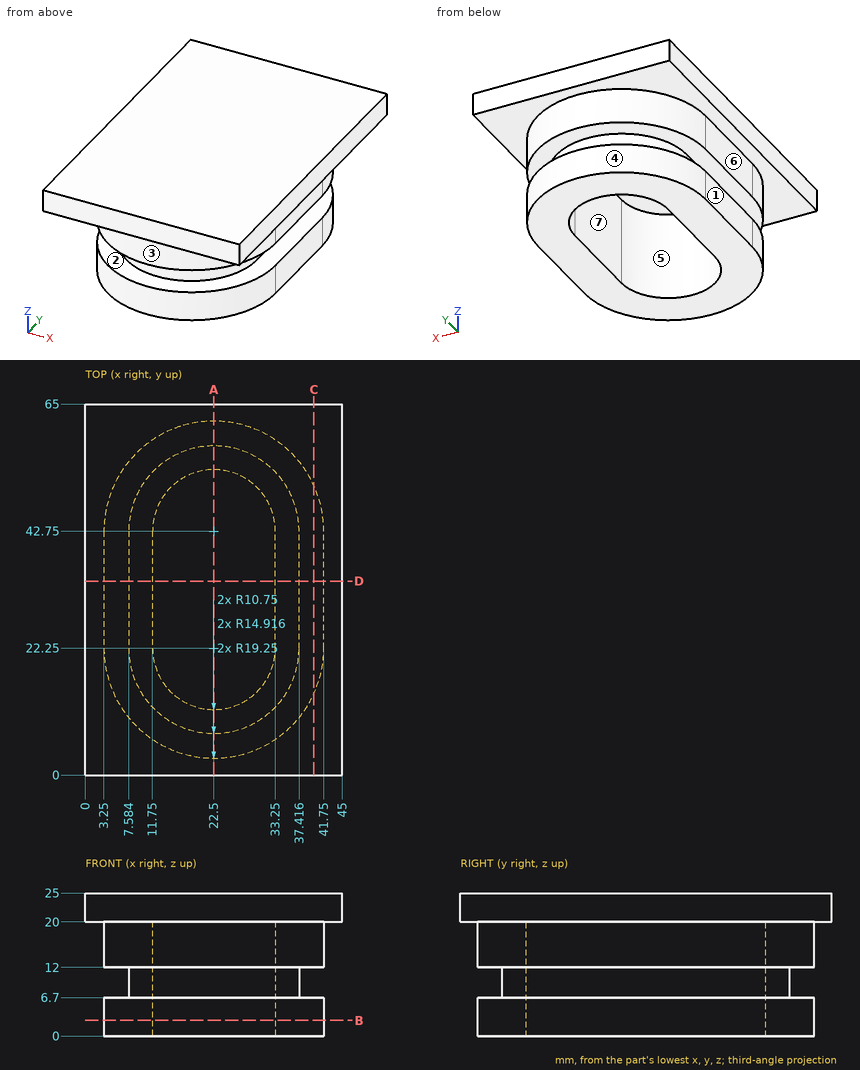
Could you check a few things on this drawing? It's one solid part, dimensions in mm from its lowest x, y, z. A direction names the side the tool comes from. Give positions to 0.01 mm unless a question says otherwise; leave off trailing zeros. Order: outer loops, then holes, each group sorted by start corner. A loop starts at its lowest first (then second) coordinate and runs counter-clockwise, first axis right, second up. Notation, with made-up numbers: (-1.75, -19.75) - (40.25, -19.75) arc R24 ccw to (40.25, -1.75) - close; hole circle Ø4 at (23, 67). An arc over 180 degrees is marked (long way). Return JSON: item names as keys, results as strings. Group by question number.
Q1. Will these pins go through, and if not, where does the flat tip stop? pin 1 Ø7.5 at (y, z) = (32, 2) entering from -X; pin 2 Ø4 at (y, z) = (34.5, 15) entering from +X; pin 3 Ø10 at (x, y) = (17, 51) entering from -Z; pin 4 Ø10 at (y, z) = (56.5, 13) entering from +X.
Q2. Thinking about a two-plate mould opening in X: for the marked faces 4, 5, 6 and 7, which applies, pulls with the +X half, pulls with the -X half, needs draft (parallel to the pull), parting line crosses it, or undercut?
Q3. Suppose I cut it at B-B, the plane z = 2.75. Please give me the cut outline in (x, y).
Q4. Suppose I cut it at C-C, the plane x = 40. Please give me the cut outline in (y, z), and give its area (3 significant figures).
Q5. Which directions (+Z, -Z, +X, -X, +Y, -Y) give clear straight access to the entire face, cutting with the end or side of a thin tool? Please do the marked faces 1, 2 and 3.
Q6. Suppose I cut it at D-D, the plane y = 34. Please give me the cut outline in (x, z), and give its area (3 significant figures).
Q7. Suppose I cut it at A-A, the plane x = 22.5. Please give me the cut outline in (y, z).
Q8. Please list where these lines run through material, in increasing order: line 1 along Y through (x, z) = (23, 16.25); line 2 along X through (y, z) = (22, 19.25). Write a range as [from, to].
Resolved:
{
 "1": {"pin 1": "stops at x = 3.25", "pin 2": "stops at x = 41.75", "pin 3": "stops at z = 0", "pin 4": "stops at x = 39.65"},
 "2": {"face 4": "parting line crosses it", "face 5": "undercut", "face 6": "pulls with the -X half", "face 7": "undercut"},
 "3": {"outline": "(3.25, 22.25) arc R19.25 ccw to (41.75, 22.25) - (41.75, 42.75) arc R19.25 ccw to (3.25, 42.75) - close; hole (11.75, 22.25) arc R10.75 ccw to (33.25, 22.25) - (33.25, 42.75) arc R10.75 ccw to (11.75, 42.75) - close"},
 "4": {"outline": "(0, 20) - (14.23, 20) - (14.23, 12) - (50.77, 12) - (50.77, 20) - (65, 20) - (65, 25) - (0, 25) - close; (14.23, 0) - (50.77, 0) - (50.77, 6.7) - (14.23, 6.7) - close", "area": "862 mm2"},
 "5": {"face 1": "-Z, -X, +Y, -Y", "face 2": "none", "face 3": "-Z, -Y"},
 "6": {"outline": "(0, 20) - (3.25, 20) - (3.25, 12) - (7.58, 12) - (7.58, 6.7) - (3.25, 6.7) - (3.25, 0) - (11.75, 0) - (11.75, 20) - (33.25, 20) - (33.25, 0) - (41.75, 0) - (41.75, 6.7) - (37.42, 6.7) - (37.42, 12) - (41.75, 12) - (41.75, 20) - (45, 20) - (45, 25) - (0, 25) - close", "area": "519 mm2"},
 "7": {"outline": "(0, 20) - (3, 20) - (3, 12) - (7.33, 12) - (7.33, 6.7) - (3, 6.7) - (3, 0) - (11.5, 0) - (11.5, 20) - (53.5, 20) - (53.5, 0) - (62, 0) - (62, 6.7) - (57.67, 6.7) - (57.67, 12) - (62, 12) - (62, 20) - (65, 20) - (65, 25) - (0, 25) - close"},
 "8": {"line 1": "y = [3.01, 11.51], [53.49, 61.99]", "line 2": "x = [3.25, 11.75], [33.25, 41.75]"}
}
